Part model, mm, in its own coordinate system. A direction names the side the tool comes from. Round coordinates to 2 decimals unless told otherwise and drop trailing zeros. Loops run counter-clockwise (first coordinate to the right, second up) from the corner with the lowest first, then second, coordinate; pieces in that order, holes last. Notation, with made-up numbers: M 71.5,65 L 94.5,65 A15 ccw 94.5,89 Z; hole C -32,38.5 d6. An arc over 180 degrees is marked long. Put each result on its own line as item: value. Start each with the question number.
1) Slice it at B-B on x = 58.5. Give the cut face in (y, z).
2) Probe line 1 along X through (y, z) = (1.75, -3); line 2 along Y through (x, z) = (-43, 0.25); line 3 along Z through (x, y) = (-44, -2). List the from-to ranges inside material, lowest first.
3) Which spindle directions (+Z, -Z, +X, -X, +Y, -Y) get a long thin tool onto all of the face, cutting with end or side? Do faces 4 (the flat face through (18, 1, 3)), 5 (the flat face through (46, -3, 0)). Say none if no direction does.
4) Drop flat-ended pins along their axis: pin 1 Ø3 at (x, z) = (-27, 3) entering from +Y; pin 2 Ø2 at (x, y) = (-17.5, 2) entering from +Z. Give the stop position or say it passes through.
5) Pull direction X, two halves, no side cores. Call faces 1 (the cylindrical face through (-0.2, 3.5, 0.1)), 2 (the flat face through (-75, 0, 0)), 3 (the flat face through (-16, 3, 1)): +X half, -X half, draft (parallel to the pull), parting line (faces both ways), or undercut.
6) Slice it at A-A on y = -1. Give the cut face in (x, z).
Autodesk Inventor part; units mm, degrees
ref_plane "Work Plane1" through (16, 0, 0) normal (1, 0, 0) x (0, 1, 0)
ref_plane "XZ Plane" through (0, 0, 0) normal (0, 1, 0) x (-1, 0, 0)
ref_plane "XY Plane" through (0, 0, 0) normal (0, 0, 1) x (1, 0, 0)
sketch "Sketch1" plane through (0, 0, 0) normal (1, 0, 0) x (0, 1, 0)
  circle A0 centre (0, 0) radius 3.5
  circle A1 centre (0, 0) radius 3
  line L0 (-3, 1.8028) -> (-3, -1.8028)
  dimension "d0" = 7
  dimension "d3" = 0.5
  dimension "d9" = 3
extrude "Extrusion1" add sketch "Sketch1" along normal mid plane 150 contours A1 | A0 L0 picked at (3.3009, 0.2732)
ref_plane "Work Plane1" through (16, 0, 0) normal (1, 0, 0) x (0, 1, 0)
extrude "Extrusion3" cut sketch "Sketch1" along normal blind 2 from surface at 16
mirror "Mirror1" about plane through (0, 0, 0) normal (1, 0, 0) of "Extrusion3"
properties part number "Linear Rod"
Recorded:
1. outline: M -3,-1.8 A3.5 ccw long -3,1.8 Z
2. line 1: x = -75 to -18, -16 to 16, 18 to 75
2. line 2: y = -3 to 3.49
2. line 3: z = -2.87 to 2.87
3. face 4: none
3. face 5: +Z, -Z, +X, -X, -Y
4. pin 1: stops at y = 3.16
4. pin 2: stops at z = 3.31
5. face 1: draft
5. face 2: -X half
5. face 3: undercut
6. outline: M -75,-3.35 L -18,-3.35 L -18,-2.83 L -16,-2.83 L -16,-3.35 L 16,-3.35 L 16,-2.83 L 18,-2.83 L 18,-3.35 L 75,-3.35 L 75,3.35 L 18,3.35 L 18,2.83 L 16,2.83 L 16,3.35 L -16,3.35 L -16,2.83 L -18,2.83 L -18,3.35 L -75,3.35 Z
